Part model, mm, in its own coordinate system. Face numbers are marked on the shaded views. A direction names the side the tool comes from. Round coordinates to 2 decimals unless told otherwise and drop trailing zeros. Loops run counter-clockwise (first coordinate to the right, second up) from the corner with the lowest first, then second, coordinate; pieces in that order, holes last.
(1) Cut at A-A on z = 5.75. List the corners of the cut face in (x, y).
(2) Tool access for the marked faces 4, 5 and 6: list every direction of +Z, -Z, +X, -X, +Y, -Y with a clear straight run to the whole face (end or side of a thin tool).
(3) Cut at C-C on x = 11. List the corners of the cut face in (y, z).
(4) Mould opens along Z. For the marked faces 1, 2 and 3 say: +Z half, -Z half, draft (parallel to the pull), parting line (faces both ways), or undercut.
(5) Probe probe 1 along X at (y, z) = (-21, 5.75); probe 2 along Z at (x, y) = (12.25, -12.25); probe 3 along Y at (x, z) = (22.25, 1.5). List the from-to ranges inside material, lowest first.
(6) Flat gauge pins, fed straight in: pin 1 (4 mm diameter, centred on x = 11, z = 10, fed in from +Y); pin 2 (2 mm diameter, centred on x = 16, z = 17.5, fed in from -Y); pin 3 (1 mm diameter, centred on y = -13, z = -1, fed in from +X); pin 4 (4 mm diameter, centred on y = 0.5, z = 17, fed in from -X). Where does each tip first touch, or does it go through?
(7) Cut at D-D on z = 11. List the corners of the cut face in (x, y).
(8) Cut at B-B on y = -6.5. List the corners of the cut face in (x, z).
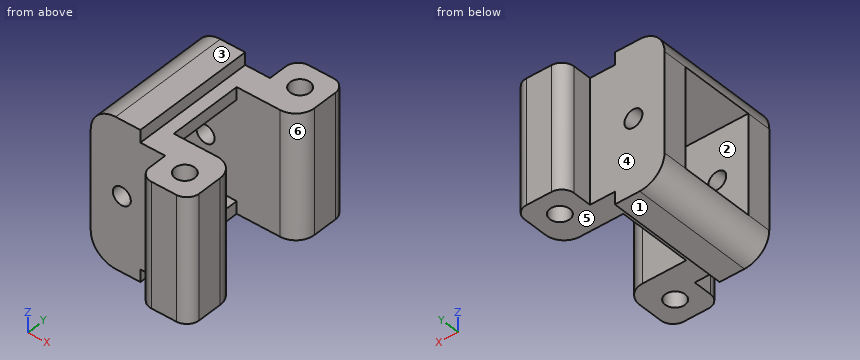
from build123d import *

# Parameters (mm, degrees)
SKETCH1_W           = 20
SKETCH1_H           = 20
BOSS_EXTRUDE1_DEPTH = 4
SKETCH2_R           = 3.7
CUT_EXTRUDE1_DEPTH  = 2.6
SKETCH3_R           = 2.1
CUT_EXTRUDE2_DEPTH  = 29.403520909
SKETCH4_W           = 12
SKETCH4_H           = 4
BOSS_EXTRUDE2_DEPTH = 12
SKETCH7_W           = 20
SKETCH7_H           = 4
BOSS_EXTRUDE3_DEPTH = 10
SKETCH8_W           = 8
SKETCH8_H           = 20
BOSS_EXTRUDE4_DEPTH = 5
SKETCH9_W           = 8
SKETCH9_H           = 20
BOSS_EXTRUDE5_DEPTH = 5
SKETCH10_R          = 1.6
CUT_EXTRUDE5_DEPTH  = 42.243181255
SKETCH11_W          = 30
SKETCH11_H          = 30
CUT_EXTRUDE6_DEPTH  = 6
SKETCH12_R          = 1.45
CUT_EXTRUDE7_DEPTH  = 42.243181255
SKETCH13_W          = 8
SKETCH13_H          = 20
BOSS_EXTRUDE6_DEPTH = 2
SKETCH14_W          = 8
SKETCH14_H          = 20
BOSS_EXTRUDE7_DEPTH = 2
SKETCH15_W          = 16
SKETCH15_H          = 12
CUT_EXTRUDE8_DEPTH  = 39.845849199
FILLET2_R           = 3
FILLET4_R           = 2
FILLET5_START       = -21
FILLET5_DEPTH       = 22


with BuildPart() as part:
    # Sketch1 → Boss-Extrude1 (new body)
    with BuildSketch(Plane(origin=(0, 0, 0), x_dir=(0, 0, -1), z_dir=(1, 0, 0))):
        with Locations((-10, -10)):
            Rectangle(SKETCH1_W, SKETCH1_H)
    extrude(amount=BOSS_EXTRUDE1_DEPTH)

    # Sketch2 → Cut-Extrude1 (cut)
    with BuildSketch(Plane(origin=(4, 0, 0), x_dir=(0, 0, -1), z_dir=(1, 0, 0))):
        with Locations((-10, -10)):
            Circle(SKETCH2_R)
    extrude(amount=-CUT_EXTRUDE1_DEPTH, mode=Mode.SUBTRACT)

    # Sketch3 → Cut-Extrude2 (cut, through all)
    with BuildSketch(Plane(origin=(1.4, 0, 0), x_dir=(0, 0, -1), z_dir=(1, 0, 0))):
        with Locations((-10, -10)):
            Circle(SKETCH3_R)
    extrude(amount=-CUT_EXTRUDE2_DEPTH, mode=Mode.SUBTRACT)

    # Sketch4 → Boss-Extrude2 (add)
    with BuildSketch(Plane(origin=(4, 0, 0), x_dir=(0, 0, -1), z_dir=(1, 0, 0))):
        Polygon((-20, 0), (-20, -20), (-16, -20), (-16, -16), (-16, -4), (-16, 0), align=None)
        with Locations((-10, -18)):
            Rectangle(SKETCH4_W, SKETCH4_H)
        Polygon((-4, -16), (-4, -20), (0, -20), (0, -4), (-4, -4), align=None)
        Polygon((0, 0), (-16, 0), (-16, -4), (-4, -4), (0, -4), align=None)
    extrude(amount=BOSS_EXTRUDE2_DEPTH)

    # Sketch7 → Boss-Extrude3 (add)
    with BuildSketch(Plane(origin=(16, 0, 0), x_dir=(0, 0, -1), z_dir=(1, 0, 0))):
        with Locations((-10, -18)):
            Rectangle(SKETCH7_W, SKETCH7_H)
        with Locations((-10, -2)):
            Rectangle(SKETCH7_W, SKETCH7_H)
    extrude(amount=BOSS_EXTRUDE3_DEPTH)

    # Sketch8 → Boss-Extrude4 (add)
    with BuildSketch(Plane(origin=(0, -20, 0), x_dir=(-1, 0, 0), z_dir=(0, -1, 0))):
        with Locations((-22, -10)):
            Rectangle(SKETCH8_W, SKETCH8_H)
    extrude(amount=BOSS_EXTRUDE4_DEPTH)

    # Sketch9 → Boss-Extrude5 (add)
    with BuildSketch(Plane(origin=(0, 0, 0), x_dir=(1, 0, 0), z_dir=(0, 1, 0))):
        with Locations((22, -10)):
            Rectangle(SKETCH9_W, SKETCH9_H)
    extrude(amount=BOSS_EXTRUDE5_DEPTH)

    # Sketch10 → Cut-Extrude5 (cut, through all)
    with BuildSketch(Plane(origin=(0, 0, 0), x_dir=(-1, 0, 0), z_dir=(0, 0, -1))):
        with Locations(Location((-22, 1, 0), (0, 0, 90))):
            Circle(SKETCH10_R)
        with Locations(Location((-22, -21, 0), (0, 0, 90))):
            Circle(SKETCH10_R)
    extrude(amount=-CUT_EXTRUDE5_DEPTH, mode=Mode.SUBTRACT)

    # Sketch11 → Cut-Extrude6 (cut)
    with BuildSketch(Plane.ZY):
        with Locations((15, -5)):
            Rectangle(SKETCH11_W, SKETCH11_H)
    extrude(amount=-CUT_EXTRUDE6_DEPTH, mode=Mode.SUBTRACT)

    # Sketch12 → Cut-Extrude7 (cut, through all)
    with BuildSketch(Plane(origin=(0, 0, 0), x_dir=(1, 0, 0), z_dir=(0, 1, 0))):
        with Locations(Location((11, -10, 0), (0, 0, 270))):
            Circle(SKETCH12_R)
    extrude(amount=-CUT_EXTRUDE7_DEPTH, mode=Mode.SUBTRACT)

    # Sketch13 → Boss-Extrude6 (add)
    with BuildSketch(Plane.XY.offset(20)):
        with Locations((10, -10)):
            Rectangle(SKETCH13_W, SKETCH13_H)
    extrude(amount=BOSS_EXTRUDE6_DEPTH)

    # Sketch14 → Boss-Extrude7 (add)
    with BuildSketch(Plane(origin=(0, 0, 0), x_dir=(-1, 0, 0), z_dir=(0, 0, -1))):
        with Locations((-10, -10)):
            Rectangle(SKETCH14_W, SKETCH14_H)
    extrude(amount=BOSS_EXTRUDE7_DEPTH)

    # Sketch15 → Cut-Extrude8 (cut, through all)
    with BuildSketch(Plane.ZY.offset(-6)):
        with Locations((10, -10)):
            Rectangle(SKETCH15_W, SKETCH15_H)
    extrude(amount=-CUT_EXTRUDE8_DEPTH, mode=Mode.SUBTRACT)

    # Fillet2
    fillet2_edges = [part.edges().sort_by_distance(p)[0] for p in [
        (26, -16, 10),
        (26, -4, 10),
    ]]
    fillet(fillet2_edges, radius=FILLET2_R)

    # Fillet4
    fillet4_edges = [part.edges().sort_by_distance(p)[0] for p in [
        (26, -25, 10),
        (18, -25, 10),
        (26, 5, 10),
        (18, 5, 10),
    ]]
    fillet(fillet4_edges, radius=FILLET4_R)

    # Fillet5: read off the stored shape, not the designer's step
    # Fillet5 outline → Fillet5 (cut)
    with BuildSketch(Plane(origin=(0, 0, 0), x_dir=(1, 0, 0), z_dir=(0, 1, 0)).offset(FILLET5_START)):
        with BuildLine():
            Line((6, 2), (6, -2))
            ThreePointArc((6, -2), (7.171572875, 0.828427125), (10, 2))
            Line((10, 2), (6, 2))
        make_face()
        with BuildLine():
            ThreePointArc((10, -22), (7.171572875, -20.828427125), (6, -18))
            Line((6, -18), (6, -22))
            Line((6, -22), (10, -22))
        make_face()
    extrude(amount=FILLET5_DEPTH, mode=Mode.SUBTRACT)


solid = part.part
Final values:
1. outline: (6, -20) - (18, -20) - (18, -23) arc R2 ccw to (20, -25) - (24, -25) arc R2 ccw to (26, -23) - (26, -19) arc R3 ccw to (23, -16) - (6, -16) - close; (6, -4) - (23, -4) arc R3 ccw to (26, -1) - (26, 3) arc R2 ccw to (24, 5) - (20, 5) arc R2 ccw to (18, 3) - (18, 0) - (6, 0) - close; hole circle Ø3.2 at (22, -21); hole circle Ø3.2 at (22, 1)
2. face 4: +Z, -Z, -X, +Y
2. face 5: -Z, +X, +Y, -Y
2. face 6: +Z, -Z, +X
3. outline: (-20, -2) - (0, -2) - (0, 8.55) - (-4, 8.55) - (-4, 2) - (-16, 2) - (-16, 8.55) - (-20, 8.55) - close; (-20, 11.45) - (-16, 11.45) - (-16, 18) - (-4, 18) - (-4, 11.45) - (0, 11.45) - (0, 22) - (-20, 22) - close
4. face 1: -Z half
4. face 2: undercut
4. face 3: +Z half
5. probe 1: x = 18 to 20.4, 23.6 to 26
5. probe 2: z = -2 to 2, 18 to 22
5. probe 3: y = -25 to -22.58, -19.42 to -16, -4 to -0.58, 2.58 to 5
6. pin 1: stops at y = 0
6. pin 2: stops at y = -20
6. pin 3: stops at x = 14
6. pin 4: stops at x = 6
7. outline: (6, -20) - (9.95, -20) - (9.95, -16) - (6, -16) - close; (6, -4) - (9.95, -4) - (9.95, 0) - (6, 0) - close; (12.05, -20) - (18, -20) - (18, -23) arc R2 ccw to (20, -25) - (24, -25) arc R2 ccw to (26, -23) - (26, -19) arc R3 ccw to (23, -16) - (12.05, -16) - close; (12.05, -4) - (23, -4) arc R3 ccw to (26, -1) - (26, 3) arc R2 ccw to (24, 5) - (20, 5) arc R2 ccw to (18, 3) - (18, 0) - (12.05, 0) - close; hole circle Ø3.2 at (22, -21); hole circle Ø3.2 at (22, 1)
8. outline: (6, 2) arc R4 ccw to (10, -2) - (14, -2) - (14, 0) - (16, 0) - (16, 2) - close; (6, 18) - (16, 18) - (16, 20) - (14, 20) - (14, 22) - (10, 22) arc R4 ccw to start
